Could you check a few things on this drawing? It's one solid part, dimensions in mm from its lowest x, y, z. A direction names the side the tool comes from. Round coordinates to 2 decimals unless told otherwise and drop trailing zeros. Write each loop counter-clockwise with the first axis right and the second up, starting at its lowest first coordinate (ties: lowest second). Pieces come first, ordered by that corner, then holes. Notation, with made-up numbers: M 32,43 L 74,43 A17 cw 74,66 Z; hole C -29.5,32 d2. An arc over 180 degrees is marked long. One line per item, written item: value. Start each with the question number.
(1) Thinking about a two-plate mould opening in X: for the marked faces 1, 2, 3 and 4, which applies, released by +X, released by -X, zero draft, split by the parting line, or undercut?
(2) I want a section at D-D on x = 164.5. Please give me the cut outline in (y, z), and give its area (3 significant figures).
(3) I'm going to push flat-ended pins straight in: pin 1 Ø8 at (y, z) = (178.5, 326.5) entering from -X; pin 2 Ø4 at (x, y) = (256.5, 159) entering from -Z; pin 3 Ø12 at (x, y) = (382, 53) entering from +Z; pin 4 Ø6 at (x, y) = (418, 122) entering from -Z. Where does each tip first touch, or does it pass through?
(4) I want a section at B-B on z = 45.5. Please give me the cut outline in (x, y) (1 decimal).
(5) I want a section at C-C on x = 418.5. Please give me the cut outline in (y, z), and give its area (3 significant figures).
(6) Which directions (+Z, -Z, +X, -X, +Y, -Y) give clear straight access to the entire face, cutting with the end or side of a thin tool? Please do the marked faces 5, 6, 7, 8 and 9.
(7) If I drill on L1, parallel to Z at x = 358, y = 26.5; L2, parallel to Z at x = 178.5, y = 112.5; L3, parallel to X at y = 61.5, z = 27 (1 decimal), over which ranges is the centre line in solid material (lowest first)?
(8) I want a section at A-A on y = 65. Please give me the cut outline in (x, z) (1 decimal), and give its area (3 significant figures).
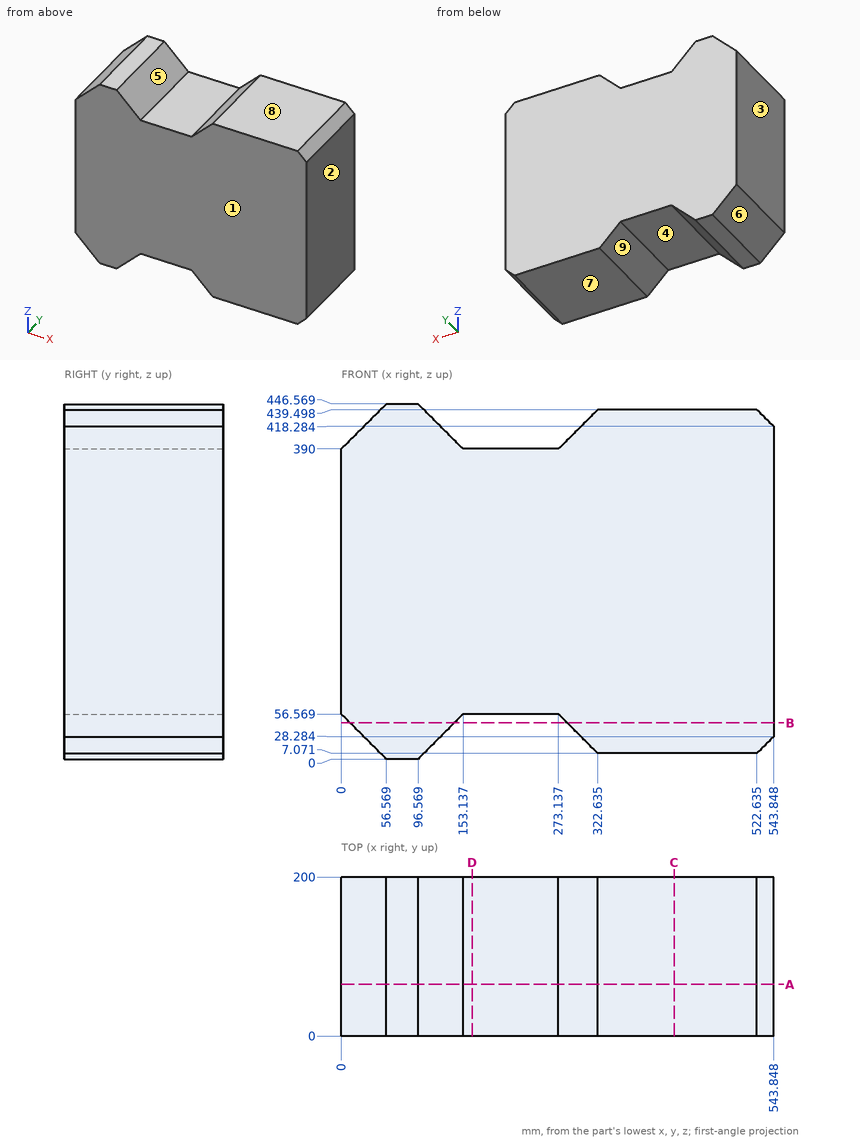
Found:
1. face 1: zero draft
1. face 2: released by +X
1. face 3: released by -X
1. face 4: undercut
2. outline: M 0,56.57 L 200,56.57 L 200,390 L 0,390 Z
2. area: 66,700 mm²
3. pin 1: stops at x = 0
3. pin 2: stops at z = 56.57
3. pin 3: stops at z = 439.5
3. pin 4: stops at z = 7.07
4. outline: M 11.1,0 L 142.1,0 L 142.1,200 L 11.1,200 Z; M 284.2,0 L 543.8,0 L 543.8,200 L 284.2,200 Z
5. outline: M 0,7.07 L 200,7.07 L 200,439.5 L 0,439.5 Z
5. area: 86,500 mm²
6. face 5: +Z, +Y, -Y
6. face 6: -Z, -X, +Y, -Y
6. face 7: -Z, +X, +Y, -Y
6. face 8: +Z, +X, +Y, -Y
6. face 9: -Z, +Y, -Y
7. L1: z = 7.07 to 439.5
7. L2: z = 56.57 to 390
7. L3: x = 29.6 to 123.6, 302.7 to 542.6
8. outline: M 0,56.6 L 56.6,0 L 96.6,0 L 153.1,56.6 L 273.1,56.6 L 322.6,7.1 L 522.6,7.1 L 543.8,28.3 L 543.8,418.3 L 522.6,439.5 L 322.6,439.5 L 273.1,390 L 153.1,390 L 96.6,446.6 L 56.6,446.6 L 0,390 Z
8. area: 216,000 mm²
